Read the model definition and answer for the solid it produces. Units are mm, in the model's axes. Face numbers are marked on the shaded views. A direction names the side the tool comes from. Coordinates: 2 decimals unless noted, no trailing zeros. Loops run counter-clockwise (first coordinate to the right, second up) from the corner with the lowest first, then second, coordinate; pieces in that order, holes last.
Q1. Which of the six approach directions +Z, -Z, +X, -X, +Y, -Y give full straight-line access (tool end or side, diameter ignored) to the marked faces 5, 6 and 7?
Q2. Flat-ended cylindrical pins translate along their axes: P1, Ø2, axis at y = -11.5, z = -2, coming from the -X side; P2, Ø1.7, axis at x = 0, y = -36, coming from the -Z side (3 decimals); P3, Ø1.5, axis at y = -11.5, z = -2, coming from the +X side. Find the tip coordinate at first contact, or state that the pin passes through.
Q3. Section A-A (x = 0.5) is taken. Give the vertices of the cut face in (y, z) (3 decimals).
Q4. The mould has two halves that part along Y. Classify the marked faces 1, 2, 3 and 4: pulls with the +Y half, pulls with the -Y half, needs draft (parallel to the pull), parting line crosses it, or undercut.
Q5. Section C-C (z = 4) is taken. Give the vertices of the cut face in (x, y).
Q6. Section D-D (x = -2) is taken. Give the vertices of the cut face in (y, z).
Q7. Straight lines are drawn through the part: line 1 (Y direction, x = 1, z = -1.5); line 2 (Y direction, x = 0.2, z = 0); line 3 (Y direction, x = 2, z = 1). For each, find the intervals that lie inside material, in ascending order.
Q8. Section B-B (y = -26) is taken. Give the vertices of the cut face in (x, z) (1 decimal).
from build123d import *

# Parameters (mm, degrees)
SKETCH2_R           = 4.7625
BOSS_EXTRUDE2_DEPTH = 12.7
SKETCH3_R           = 1.5875
BOSS_EXTRUDE3_DEPTH = 19.05
SKETCH4_W           = 6.35
SKETCH4_H           = 6.35
SKETCH4_R           = 1.190625
BOSS_EXTRUDE4_DEPTH = 1.5875
FILLET2_R           = 0.508


with BuildPart() as part:
    # Sketch2 → Boss-Extrude2 (new body)
    with BuildSketch(Plane(origin=(0, 0, 0), x_dir=(1, 0, 0), z_dir=(0, 1, 0))):
        with Locations(Location((0, 0, 0), (0, 0, 270))):
            Circle(SKETCH2_R)
    extrude(amount=-BOSS_EXTRUDE2_DEPTH)

    # Sketch3 → Boss-Extrude3 (add)
    with BuildSketch(Plane.XZ.offset(12.7)):
        with Locations(Location((0, 0, 0), (0, 0, 90))):
            Circle(SKETCH3_R)
    extrude(amount=BOSS_EXTRUDE3_DEPTH)

    # Sketch4 → Boss-Extrude4 (add, symmetric)
    with BuildSketch(Plane(origin=(0, 0, 0), x_dir=(0, 0, -1), z_dir=(1, 0, 0))):
        with Locations((0, -34.925)):
            Rectangle(SKETCH4_W, SKETCH4_H)
        with Locations((0, -34.925)):
            Circle(SKETCH4_R, mode=Mode.SUBTRACT)
    extrude(amount=BOSS_EXTRUDE4_DEPTH, both=True)

    # Fillet2
    fillet2_edges = [part.edges().sort_by_distance(p)[0] for p in [
        (1.5875, -34.925, 3.175),
        (1.5875, -34.925, -3.175),
        (-1.5875, -34.925, 3.175),
        (-1.5875, -34.925, -3.175),
    ]]
    fillet(fillet2_edges, radius=FILLET2_R)


solid = part.part
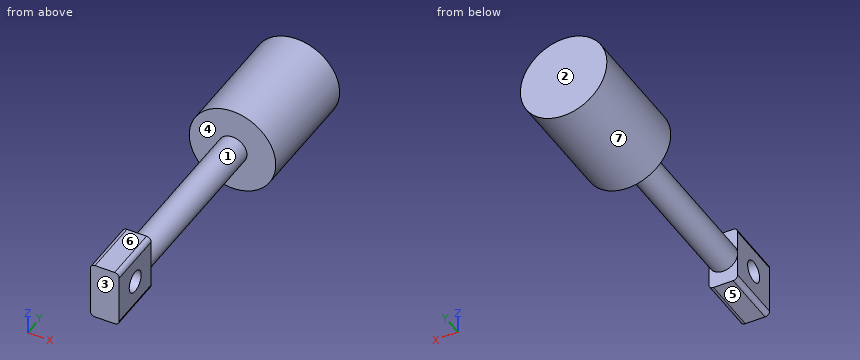
Numbers:
1. face 5: -Z, +X, -X, -Y
1. face 6: +Z, +X, -X, -Y
1. face 7: +Y, -Y
2. P1: stops at x = -4.66
2. P2: stops at z = -3.175
2. P3: stops at x = 4.6
3. outline: (-38.1, -3.175) - (-31.75, -3.175) - (-31.75, -1.507) - (-12.7, -1.507) - (-12.7, -4.736) - (0, -4.736) - (0, 4.736) - (-12.7, 4.736) - (-12.7, 1.507) - (-31.75, 1.507) - (-31.75, 3.175) - (-38.1, 3.175) - close; hole circle Ø2.381 at (-34.925, 0)
4. face 1: undercut
4. face 2: pulls with the +Y half
4. face 3: pulls with the -Y half
4. face 4: undercut
5. outline: (-2.58, -12.7) - (2.58, -12.7) - (2.58, 0) - (-2.58, 0) - close
6. outline: (-12.7, -4.32) - (0, -4.32) - (0, 4.32) - (-12.7, 4.32) - close
7. line 1: y = -38.1 to -31.75, -12.7 to 0
7. line 2: y = -38.1 to -36.12, -33.73 to 0
7. line 3: y = -12.7 to 0
8. outline: circle Ø3.2 at (0, 0)
